Model file for the job. Use its own axes, mm. Face numbers are marked on the shaded views. A direction names the side the tool comes from. Round coordinates to 2 decimals unless told otherwise and drop trailing zeros. Loops run counter-clockwise (first coordinate to the right, second up) from the corner with the lowest first, then second, coordinate; pieces in that order, holes last. Notation, with made-up numbers: (-33.5, -32.75) - (1.5, -32.75) arc R25 cw to (1.5, 1.25) - close; hole circle Ø3 at (73, 88.25). An arc over 180 degrees is marked (long way). Use one line per item in the form item = value.
Autodesk Inventor part; units mm, degrees
ref_plane "YZ Plane" through (0, 0, 0) normal (1, 0, 0) x (0, 1, 0)
ref_plane "XZ Plane" through (0, 0, 0) normal (0, 1, 0) x (-1, 0, 0)
ref_plane "XY Plane" through (0, 0, 0) normal (0, 0, 1) x (1, 0, 0)
sketch "Sketch3" plane through (0, 0, 0) normal (1, 0, 0) x (0, 1, 0)
  circle A0 centre (0, 0) radius 15.875 construction
  circle A1 centre (0, 0) radius 14.6304
  dimension "d8" = 31.75
  dimension "d9" = 1.2446
extrude "Extrusion3" add sketch "Sketch3" along normal blind 12.7
sketch "Sketch4" plane through (12.7, 0, 0) normal (1, 0, 0) x (0, 0, -1)
  circle A0 centre (0, 0) radius 4.7625
  dimension "d12" = 9.525
extrude "Extrusion4" add sketch "Sketch4" along normal blind 31.75
sketch "Sketch5" plane through (44.45, 0, 0) normal (1, 0, 0) x (0, 0, -1)
  circle A0 centre (0, 0) radius 2.4892
  dimension "d15" = 4.9784
extrude "Extrusion5" cut sketch "Sketch5" against normal blind 25.4
sketch "Sketch6" plane through (0, 0, 0) normal (-1, 0, 0) x (0, 0, 1)
  circle A0 centre (0, 0) radius 9.525
  dimension "d18" = 19.05
extrude "Extrusion6" cut sketch "Sketch6" against normal blind 9.525
properties part number "Long roller plug"
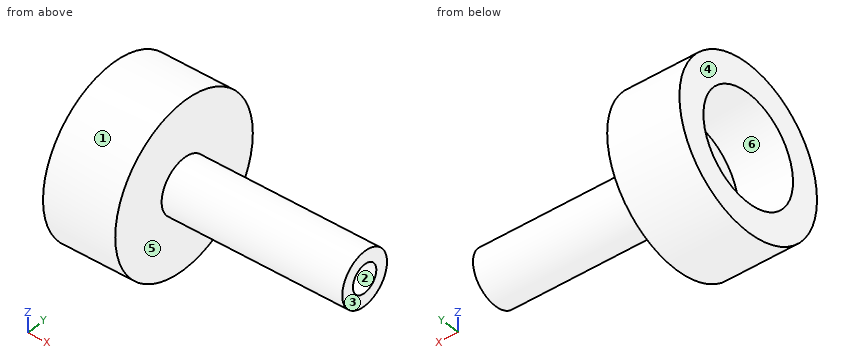
1. Wall check: probe 1 along X at (y, z) = (-5.5, 3) (3 decimals); probe 2 along X at (y, z) = (-2.25, -2.75) (3 decimals); probe 3 along Z at (x, y) = (25, -1.75). Give the ranges that are in metal, low to high.
Geometry check:
probe_1 = 9.525 to 12.7
probe_2 = 9.525 to 44.45
probe_3 = -4.43 to -1.77, 1.77 to 4.43
2. Tool access for the marked faces 4, 5 and 6: list every direction of +Z, -Z, +X, -X, +Y, -Y with a clear straight run to the whole face (end or side of a thin tool).
Geometry check:
face_4 = +Z, -Z, -X, +Y, -Y
face_5 = +X
face_6 = -X
3. Cut at C-C, the plane x = 7.5. Give the cut face in (y, z) (3 decimals).
Geometry check:
outline = circle Ø29.261 at (0, 0); hole circle Ø19.05 at (0, 0)
4. Flat gauge pins, fed straight in: pin 1 (3 mm diameter, centred on y = 7, z = 10.5, fed in from +X); pin 2 (5.5 mm diameter, centred on y = 0, z = 0, fed in from +X); pin 3 (10 mm diameter, centred on x = 22, z = -6, fed in from +Y); pin 4 (8 mm diameter, centred on x = 23, z = -10, fed in from +Y). Where does each tip first touch, or does it go through?
Geometry check:
pin_1 = 12.7
pin_2 = 44.45
pin_3 = 4.66
pin_4 = through
5. Pull direction Z, two halves, no side cores. Call the marked faces 1, 2 and 3: +Z half, -Z half, draft (parallel to the pull), parting line (faces both ways), or undercut.
Geometry check:
face_1 = parting line
face_2 = undercut
face_3 = draft
6. Cut at D-D, the plane x = 16.5. Give the cut face in (y, z) (1 decimal), plus the area to 3 significant figures.
Geometry check:
outline = circle Ø9.5 at (0, 0)
area = 71.3 mm^2
